```python
from build123d import *

# Parameters (mm, degrees)
SKETCH1_R           = 50
BOSS_EXTRUDE1_DEPTH = 7.5
SKETCH2_R           = 75
BOSS_EXTRUDE2_DEPTH = 7.5
SKETCH3_W           = 10
SKETCH3_H           = 60
BOSS_EXTRUDE3_DEPTH = 150
FILLET1_R           = 30
FILLET2_R           = 10
CUT_EXTRUDE1_DEPTH  = 10
FILLET3_R           = 2.5
SKETCH5_R           = 9
CUT_EXTRUDE6_DEPTH  = 212.960382158


# Some blends are built 0.0001 mm under size
with BuildPart() as part:
    # Sketch1 → Boss-Extrude1 (new body)
    with BuildSketch(Plane(origin=(0, 0, 0), x_dir=(1, 0, 0), z_dir=(0, 1, 0))):
        with Locations(Location((0, 0, 0), (0, 0, 270))):
            Circle(SKETCH1_R)
    extrude(amount=BOSS_EXTRUDE1_DEPTH)

    # Sketch2 → Boss-Extrude2 (add)
    with BuildSketch(Plane(origin=(0, 7.5, 0), x_dir=(1, 0, 0), z_dir=(0, 1, 0))):
        with Locations(Location((0, 0, 0), (0, 0, 270))):
            Circle(SKETCH2_R)
    extrude(amount=BOSS_EXTRUDE2_DEPTH)

    # Sketch3 → Boss-Extrude3 (add)
    with BuildSketch(Plane(origin=(0, 15, 0), x_dir=(1, 0, 0), z_dir=(0, 1, 0))):
        with Locations((29.896331169, 0)):
            Rectangle(SKETCH3_W, SKETCH3_H)
        with Locations((-29.896331169, 0)):
            Rectangle(SKETCH3_W, SKETCH3_H)
    extrude(amount=BOSS_EXTRUDE3_DEPTH)

    # Fillet1
    fillet1_edges = [part.edges().sort_by_distance(p)[0] for p in [
        (29.896331169, 165, 30),
        (-29.896331169, 165, 30),
        (-29.896331169, 165, -30),
        (29.896331169, 165, -30),
    ]]
    fillet(fillet1_edges, radius=FILLET1_R - 0.0001)  # a hair under: the kernel refuses the full size

    # Fillet2
    # the kernel refuses this fillet: 10 mm, written as the material it takes off along each edge
    with BuildSketch(Plane(origin=(0, 15, 0), x_dir=(0, 0, 1), z_dir=(-1, 0, 0))) as fillet2_piece_1:
        with BuildLine():
            CenterArc((65.317541634, -10), FILLET2_R, 14.477512186, 75.522487814)
            Line((75, -7.5), (75.193649167, -7.45))
            ThreePointArc((75.193649167, -7.45), (75.2, -3.75), (75.2, 0))
            Line((75.2, 0), (75, 0.2))
            Line((75, 0.2), (65.317541634, 0.2))
            Line((65.317541634, 0.2), (65.317541634, 0))
        make_face()
    revolve(axis=Axis((0, 15, 0), (0, 1, 0)), mode=Mode.SUBTRACT)

    # Sketch4 → Cut-Extrude1 (cut)
    with BuildSketch(Plane(origin=(34.896331169, 0, 0), x_dir=(0, 0, -1), z_dir=(1, 0, 0))):
        with BuildLine():
            Line((-11.15, 195), (11.15, 195))
            Line((11.15, 195), (11.15, 140))
            ThreePointArc((11.15, 140), (9.685533906, 136.464466094), (6.15, 135))
            Line((6.15, 135), (-6.15, 135))
            ThreePointArc((-6.15, 135), (-9.685533906, 136.464466094), (-11.15, 140))
            Line((-11.15, 140), (-11.15, 195))
        make_face()
    extrude(amount=-CUT_EXTRUDE1_DEPTH, mode=Mode.SUBTRACT)

    # Fillet3
    fillet3_edges = [part.edges().sort_by_distance(p)[0] for p in [
        (29.896331169, 162.851019733, 11.15),
        (29.896331169, 162.851019733, -11.15),
    ]]
    fillet(fillet3_edges, radius=FILLET3_R)

    # Sketch5 → Cut-Extrude6 (cut, through all)
    with BuildSketch(Plane(origin=(34.896331169, 0, 0), x_dir=(0, 0, -1), z_dir=(1, 0, 0))):
        with Locations((0, 146)):
            Circle(SKETCH5_R)
    extrude(amount=-CUT_EXTRUDE6_DEPTH, mode=Mode.SUBTRACT)


solid = part.part
```
Geometry check sheet. Reference: the model listing, model coordinates, mm. A direction names the side the tool comes from. Round coordinates to 2 decimals unless told otherwise and drop trailing zeros. Order: outer loops, then holes, each group sorted by start corner. A loop starts at its lowest first (then second) coordinate and runs counter-clockwise, first axis right, second up. Notation, with made-up numbers: (-9.75, -35.75) - (18.25, -35.75) arc R17 cw to (18.25, -24.75) - close; hole circle Ø10 at (-13.5, 7.5). An arc over 180 degrees is marked (long way). Use a Markdown table: item, result. Add a question column.
1) Section check C-C (y = 146). Record the cut outline in (x, z), then the cut area to 3 significant figures.
2) Section check B-B (x = 0). Record the cut outline in (y, z).
3) Section check A-A (y = 121). Record the cut outline in (x, z).
4) Set-up check for faces 4 (the cylindrical face through (15.02, 3.7, 47.69)), 5 (the cylindrical face through (29.97, 136.43, 9.65)), 6 (the flat face through (-30, 74, 30)), 7 (the flat face through (-24.896, 89, 0)), 8 (the flat face through (34.896, 87, 0)): record each of +Z, -Z, +X, -X, +Y, -Y from which the full face is reachable in a straight line by a thin tool's end or side.
5) Thickness scan on line 1 along Y through (x, z) = (-26.75, 0); line 2 along X through (y, z) = (93, 17); line 3 along Y through (x, z) = (3.5, -57). Record the ranges inside material, lowest first.
6) Gauge pin test, flat ends, axial feed: P1, Ø3, axis at x = -31, y = 93.5, coming from the -Z side; P2, Ø2, axis at y = 144.5, z = -17.5, coming from the -X side; P3, Ø3, axis at x = 32.5, z = -3, coming from the +Y side. Record the tip position at first contact, or that the pin passes through.
7) Mould release check, pull along X, two halves, no side actions. Record for faces 1 (the flat face through (1, 15, -1)), 2 (the flat face through (-34.896, 89, 0)), 3 (the cylindrical face through (-29.826, 154.923, 1.172)): released by +X, released by -X, zero draft, split by the parting line, or undercut.
Established:
| question | item | result |
|---|---|---|
| 1 | outline | (-34.9, -27.91) - (-24.9, -27.91) - (-24.9, -9) - (-34.9, -9) - close; (-34.9, 9) - (-24.9, 9) - (-24.9, 27.91) - (-34.9, 27.91) - close; (24.9, -27.91) - (34.9, -27.91) - (34.9, -11.15) - (24.9, -11.15) - close; (24.9, 11.15) - (34.9, 11.15) - (34.9, 27.91) - (24.9, 27.91) - close |
| 1 | area | 713 mm2 |
| 2 | outline | (0, -50) - (7.5, -50) - (7.5, -75) arc R10 ccw to (15, -65.32) - (15, 65.32) arc R10 ccw to (7.5, 75) - (7.5, 50) - (0, 50) - close |
| 3 | outline | (-34.9, -30) - (-24.9, -30) - (-24.9, 30) - (-34.9, 30) - close; (24.9, -30) - (34.9, -30) - (34.9, 30) - (24.9, 30) - close |
| 4 | face 4 | -Y |
| 4 | face 5 | +X, +Y |
| 4 | face 6 | +Z, +X, -X, +Y |
| 4 | face 7 | +Z, -Z, +Y |
| 4 | face 8 | +Z, -Z, +X, +Y |
| 5 | line 1 | 0 to 137, 155 to 165 |
| 5 | line 2 | -34.9 to -24.9, 24.9 to 34.9 |
| 5 | line 3 | 7.5 to 15 |
| 6 | P1 | z = -30 |
| 6 | P2 | x = -34.9 |
| 6 | P3 | y = 135 |
| 7 | face 1 | undercut |
| 7 | face 2 | released by -X |
| 7 | face 3 | zero draft |
